The figure shows three views and two pictorial views of one solid part (mm, origin at its lowest corner). Answer the questions. A direction names the side the tool comes from. Coordinates: 2 decimals unless noted, no trailing zeros. Loops run counter-clockwise (first coordinate to the right, second up) from the corner with the lowest first, then second, coordinate; pieces in that order, holes last. Notation, with made-up numbers: (48.25, 37.5) - (97.25, 37.5) arc R13 ccw to (97.25, 46.5) - close; hole circle Ø4 at (-19.5, 42.5). An arc over 180 degrees is marked (long way). Return JSON: item names as keys, results as strings. Group by question number.
1. Each of these flat-tipped pins is pushed along its axis until it touches: P1, Ø6.5, axis at y = 7.5, z = 30, coming from the -X side; P2, Ø11.5, axis at x = 75, y = 37.5, coming from the -Z side; P3, Ø2, axis at y = 8, z = 29.5, coming from the -X side. Where does it stop, or does it pass through?
2. Section A-A (z = 30) is taken. Write down the section's boundary in (x, y), and give its area (3 significant figures).
3. Section C-C (y = 7.5) is taken. Write down the section's boundary in (x, z), and give its area (3 significant figures).
4. Find the intervals of material crossed by line 1 along X through (y, z) = (111.3, 30); line 2 along Y through (x, z) = (77, 30); line 3 along X through (y, z) = (57, 28.5), in increasing order.
5. Section B-B (x = 43) is taken. Write down the section's boundary in (y, z).
6. Section D-D (x = 67.5) is taken. Write down the section's boundary in (y, z), and give its area (3 significant figures).
7. Which of the six approach directions +Z, -Z, +X, -X, +Y, -Y give full straight-line access (tool end or side, diameter ignored) to the marked faces 1 and 2?
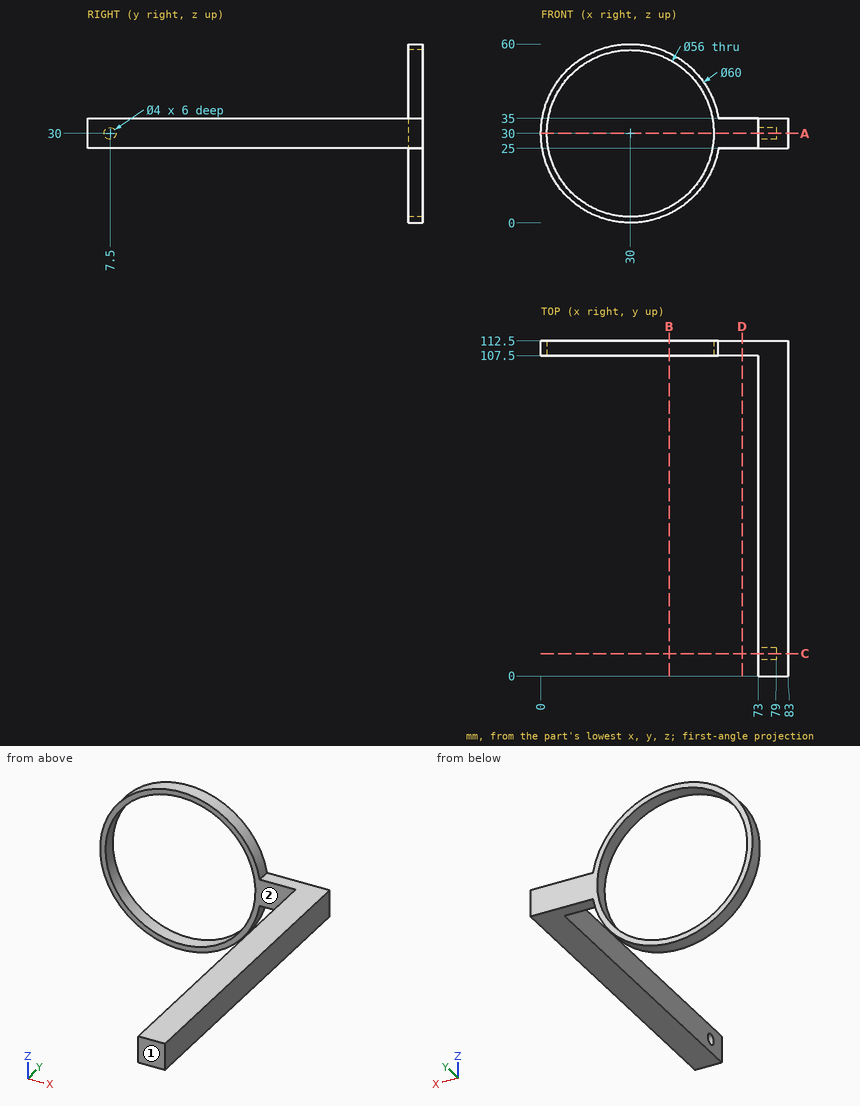
The answers:
{
 "1": {"P1": "stops at x = 73", "P2": "stops at z = 25", "P3": "stops at x = 79"},
 "2": {"outline": "(0, 107.5) - (2, 107.5) - (2, 112.5) - (0, 112.5) - close; (58, 107.5) - (73, 107.5) - (73, 9.5) - (79, 9.5) - (79, 5.5) - (73, 5.5) - (73, 0) - (83, 0) - (83, 112.5) - (58, 112.5) - close", "area": "1,190 mm2"},
 "3": {"outline": "(73, 25) - (83, 25) - (83, 35) - (73, 35) - (73, 32) - (79, 32) - (79, 28) - (73, 28) - close", "area": "76.0 mm2"},
 "4": {"line 1": "x = 0 to 2, 58 to 83", "line 2": "y = 0 to 5.5, 9.5 to 112.5", "line 3": "x = 73 to 83"},
 "5": {"outline": "(107.5, 2.96) - (112.5, 2.96) - (112.5, 5.2) - (107.5, 5.2) - close; (107.5, 54.8) - (112.5, 54.8) - (112.5, 57.04) - (107.5, 57.04) - close"},
 "6": {"outline": "(107.5, 25) - (112.5, 25) - (112.5, 35) - (107.5, 35) - close", "area": "50.0 mm2"},
 "7": {"face 1": "+Z, -Z, +X, -X, -Y", "face 2": "+Z, -Z, -X, -Y"}
}
